Work out the finished part from the listing and answer in its coordinate system (mm). Give positions to 0.01 mm unless a question says otherwise; leave off trailing zeros. Write each loop counter-clockwise with the first axis right and the second up, starting at its lowest first coordinate (ties: lowest second). Pieces come first, ordered by that corner, then holes. Notation, with made-up numbers: (50, -19) -> (81, -19) arc R20 ccw to (81, 12) -> close; hole circle Ø2 at (13, 34). An arc over 180 degrees is marked (long way). Use a Markdown table: item, result. Add a question column.
Q1. Consider line 1 (Y direction, x = 0, z = -81) (3 decimals); line 2 (X direction, y = 1, z = -145); line 3 (X direction, y = -0.75, z = -47). Determine where each line is inside the solid, lowest interval first.
Q2. Section B-B, the plane z = -119.5 is taken. Give the vertices of the cut face in (x, y) (3 decimals).
Q3. Each of these flat-tipped pins is pushed along its axis until it touches: pin 1 Ø4.5 at (x, y) = (0, 0) entering from +Z; pin 2 Ø6 at (y, z) = (-3, -104) entering from +X. Where does it stop, or does it pass through?
Q4. Section A-A, the plane y = 0 is taken. Give the vertices of the cut face in (x, z) (3 decimals).
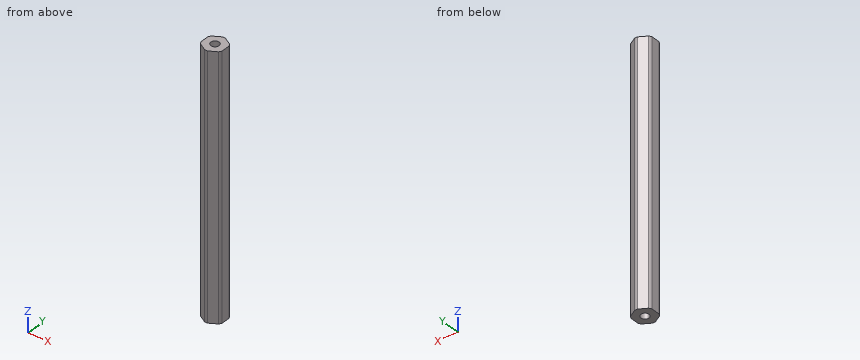
from build123d import *

# Parameters (mm, degrees)
SKETCH2_R           = 2.4892
BOSS_EXTRUDE1_DEPTH = 155.575


with BuildPart() as part:
    # Sketch2 → Boss-Extrude1 (new body)
    with BuildSketch(Plane.XY):
        with BuildLine():
            Line((-0.893039494, 6.816751826), (-5.456960506, 4.181770802))
            ThreePointArc((-5.456960506, 4.181770802), (-5.953924651, 3.4375), (-6.35, 2.634981025))
            Line((-6.35, 2.634981025), (-6.35, -2.634981025))
            ThreePointArc((-6.35, -2.634981025), (-5.953924651, -3.4375), (-5.456960506, -4.181770802))
            Line((-5.456960506, -4.181770802), (-0.893039494, -6.816751826))
            ThreePointArc((-0.893039494, -6.816751826), (0, -6.875), (0.893039494, -6.816751826))
            Line((0.893039494, -6.816751826), (5.456960506, -4.181770802))
            ThreePointArc((5.456960506, -4.181770802), (5.953924651, -3.4375), (6.35, -2.634981025))
            Line((6.35, -2.634981025), (6.35, 2.634981025))
            ThreePointArc((6.35, 2.634981025), (5.953924651, 3.4375), (5.456960506, 4.181770802))
            Line((5.456960506, 4.181770802), (0.893039494, 6.816751826))
            ThreePointArc((0.893039494, 6.816751826), (0, 6.875), (-0.893039494, 6.816751826))
        make_face()
        Circle(SKETCH2_R, mode=Mode.SUBTRACT)
    extrude(amount=-BOSS_EXTRUDE1_DEPTH)


solid = part.part
Result set:
| question | item | result |
|---|---|---|
| 1 | line 1 | y = -6.875 to -2.489, 2.489 to 6.875 |
| 1 | line 2 | x = -6.35 to -2.28, 2.28 to 6.35 |
| 1 | line 3 | x = -6.35 to -2.37, 2.37 to 6.35 |
| 2 | outline | (-6.35, -2.635) arc R6.875 ccw to (-5.457, -4.182) -> (-0.893, -6.817) arc R6.875 ccw to (0.893, -6.817) -> (5.457, -4.182) arc R6.875 ccw to (6.35, -2.635) -> (6.35, 2.635) arc R6.875 ccw to (5.457, 4.182) -> (0.893, 6.817) arc R6.875 ccw to (-0.893, 6.817) -> (-5.457, 4.182) arc R6.875 ccw to (-6.35, 2.635) -> close; hole circle Ø4.978 at (0, 0) |
| 3 | pin 1 | passes through |
| 3 | pin 2 | stops at x = 6.35 |
| 4 | outline | (-6.35, -155.575) -> (-2.489, -155.575) -> (-2.489, 0) -> (-6.35, 0) -> close; (2.489, -155.575) -> (6.35, -155.575) -> (6.35, 0) -> (2.489, 0) -> close |
